Work out the finished part from the listing and answer in its coordinate system (mm). A direction names the side the tool comes from. Give positions to 0.01 mm unless a question says otherwise; leave off trailing zeros. Loops run counter-clockwise (first coordinate to the right, second up) from the corner with the lowest first, then second, coordinate; pieces in that order, holes last. Notation, with made-up numbers: (79, 63) - (126, 63) arc R20 ccw to (126, 91) - close; hole circle Ø1 at (0, -21). An arc over 180 degrees is marked (long way). One line per item, written item: value.
from build123d import *

# Parameters (mm, degrees)
F1_DEPTH = 3
F2_R     = 5


with BuildPart() as f1:
    # F0 (on Top) → F1 (new body)
    with BuildSketch(Plane.XY):
        with BuildLine():
            Line((-50.5, 0), (64.696152, 0))
            Line((64.696152, 0), (64.696152, 41.358293))
            Line((64.696152, 41.358293), (0, 41.358293))
            Line((0, 41.358293), (0, 46.358293))
            ThreePointArc((0, 46.358293), (-6, 52.358293), (-12, 46.358293))
            Line((-12, 46.358293), (-12, 37))
            Line((-12, 37), (-50.5, 37))
            Line((-50.5, 37), (-50.5, 31))
            Line((-50.5, 31), (-20.5, 31))
            Line((-20.5, 31), (-20.5, 25))
            Line((-20.5, 25), (-12, 25))
            Line((-12, 25), (-12, 28.5))
            Line((-12, 28.5), (0, 28.5))
            Line((0, 28.5), (10, 28.5))
            Line((10, 28.5), (10, 8.5))
            Line((10, 8.5), (0, 8.5))
            Line((0, 8.5), (-12, 8.5))
            Line((-12, 8.5), (-12, 12))
            Line((-12, 12), (-20.5, 12))
            Line((-20.5, 12), (-20.5, 6))
            Line((-20.5, 6), (-50.5, 6))
            Line((-50.5, 6), (-50.5, 0))
        make_face()
    extrude(amount=F1_DEPTH)

    # F2
    f2_edges = [f1.edges().sort_by_distance(p)[0] for p in [
        (64.696152, 0, 1.5),
    ]]
    fillet(f2_edges, radius=F2_R)


solid = f1.part
1. For faces 4 (the flat face through (33, 41.358, 1)), 5 (the flat face through (-35, 6, 1)), 6 (the flat face through (10, 19, 1)), determine the directions among +Z, -Z, +X, -X, +Y, -Y from which every point of the face is accessible in a straight line to the end or side of a thin tool.
Output:
face 4: +Z, -Z, +X, +Y
face 5: +Z, -Z, -X
face 6: +Z, -Z
2. Section B-B (z = 2) is taken. Write down the section's boundary in (x, y), and give its area (3 significant figures).
Output:
outline: (-50.5, 0) - (59.7, 0) arc R5 ccw to (64.7, 5) - (64.7, 41.36) - (0, 41.36) - (0, 46.36) arc R6 ccw to (-12, 46.36) - (-12, 37) - (-50.5, 37) - (-50.5, 31) - (-20.5, 31) - (-20.5, 25) - (-12, 25) - (-12, 28.5) - (10, 28.5) - (10, 8.5) - (-12, 8.5) - (-12, 12) - (-20.5, 12) - (-20.5, 6) - (-50.5, 6) - close
area: 3,410 mm²
3. The mould has two halves that part along Y. Classify faces 1 (the cylindrical face through (-5.868, 52.357, 1.479)), 2 (the flat face through (64.696, 23, 1)), 3 (the flat face through (-1, 28.5, 1)): released by +Y, released by -Y, zero draft, split by the parting line, or undercut.
Output:
face 1: released by +Y
face 2: zero draft
face 3: undercut
4. Section C-C (y = 17.5) is taken. Write down the section's boundary in (x, z).
Output:
outline: (10, 0) - (64.7, 0) - (64.7, 3) - (10, 3) - close
5. Find the intervals of material crossed by line 1 along Y through (x, z) = (-16.5, 2.9); line 2 along X through (y, z) = (10, 0.65); line 3 along Y through (x, z) = (-22, 1.4), in increasing order.
Output:
line 1: y = 0 to 12, 25 to 37
line 2: x = -20.5 to -12, 10 to 64.7
line 3: y = 0 to 6, 31 to 37
6. Section D-D (x = 25.5) is taken. Write down the section's boundary in (y, z).
Output:
outline: (0, 0) - (41.36, 0) - (41.36, 3) - (0, 3) - close
7. Section A-A (x = -6) is taken. Write down the section's boundary in (y, z), and give its area (3 significant figures).
Output:
outline: (0, 0) - (8.5, 0) - (8.5, 3) - (0, 3) - close; (28.5, 0) - (52.36, 0) - (52.36, 3) - (28.5, 3) - close
area: 97.1 mm²
8. Flat-ended cylindrical pins translate along their axes: pin 1 Ø0.9 at (y, z) = (27, 1) entering from -X; pin 2 Ø0.9 at (x, z) = (2.5, 2) entering from +Y; pin 3 Ø0.9 at (y, z) = (43, 1) entering from +X; pin 4 Ø5 at (x, y) = (19, 22.5) entering from -Z. Find the tip coordinate at first contact, or state that the pin passes through.
Output:
pin 1: stops at x = -20.5
pin 2: stops at y = 41.36
pin 3: stops at x = 0
pin 4: stops at z = 0
